from build123d import *

# Parameters (mm, degrees)
F0_W     = 50
F0_H     = 200
F1_DEPTH = 10
F2_R     = 3
F3_DEPTH = 25
F5_DEPTH = 25
F6_W     = 10
F6_H     = 10
F7_DEPTH = 10


with BuildPart() as f1:
    # F0 (on Front) → F1 (new body)
    with BuildSketch(Plane.XZ):
        Rectangle(F0_W, F0_H)
    extrude(amount=F1_DEPTH)

    # F2 (on face) → F3 (cut)
    with BuildSketch(Plane.XZ.offset(10)):
        with Locations((0, -25)):
            Circle(F2_R)
    extrude(amount=-F3_DEPTH, mode=Mode.SUBTRACT)

    # F4 (on face) → F5 (cut)
    with BuildSketch(Plane.XZ.offset(10)):
        with BuildLine():
            Line((10, 105), (-10, 105))
            Line((-10, 105), (-10, 75))
            ThreePointArc((-10, 75), (-8.5, 73.5), (-7, 75))
            Line((-7, 75), (7, 75))
            ThreePointArc((7, 75), (8.5, 73.5), (10, 75))
            Line((10, 75), (10, 105))
        make_face()
    extrude(amount=-F5_DEPTH, mode=Mode.SUBTRACT)

    # F6 (on face) → F7 (join)
    with BuildSketch(Plane.XZ.offset(10)):
        with Locations((-30, 65)):
            Rectangle(F6_W, F6_H)
        with Locations((30, 65)):
            Rectangle(F6_W, F6_H)
        with Locations((-30, -5)):
            Rectangle(F6_W, F6_H)
        with Locations((30, -5)):
            Rectangle(F6_W, F6_H)
    extrude(amount=-F7_DEPTH)


solid = f1.part
Source: CAD feature listing. Evaluate the final solid. Frame: model axes, mm. A direction names the side the tool comes from. Coordinates: 2 decimals unless noted, no trailing zeros. Loops run counter-clockwise (first coordinate to the right, second up) from the corner with the lowest first, then second, coordinate; pieces in that order, holes last. Notation, with made-up numbers: (5.25, 45.25) -> (16.25, 45.25) arc R22 cw to (16.25, 64.25) -> close; hole circle Ø7 at (85, 7.5). An arc over 180 degrees is marked (long way). Answer in a Markdown table with one row per item. Add a question column.
Q1. Ray query, line 1 along Z through (x, y) = (0, -7.25); line 2 along X through (y, z) = (-3.5, 82); line 3 along X through (y, z) = (-3, -48). Return the intervals inside material, ascending.
Q2. Section A-A on y = -1.5. Return the cut outline in (x, z).
Q3. Section B-B on x = 0. Return the cut outline in (y, z), and give its area (3 significant figures).
Q4. Contact query for flat-ended pins moving along their axis: pin 1 Ø3 at (x, y) = (-30.5, -5) entering from -Z; pin 2 Ø1 at (y, z) = (-2.5, 44.5) entering from +X; pin 3 Ø5 at (x, z) = (0, -25) entering from +Y; pin 4 Ø5 at (y, z) = (-3, 81.5) entering from -X. Output: stop coordinate, or through.
Q5. Reachability of faces 5 (the face through (25, -5, -56)), 6 (the face through (-30, -5, 70)), 7 (the face through (30, -5, 0)), 8 (the face through (0, -5, 75)) from +Z, -Z, +X, -X, +Y, -Y: full face, straight path, thin tool, end or side. Return the list, or none.
Q6. Section D-D on z = 5.5. Return the cut outline in (x, y), and give its area (3 significant figures).
Q7. Section C-C on z = -25. Return the cut outline in (x, y), and give its area (3 significant figures).
Q8. Pull-direction query (Z, two-part tool) for faces 1 (the face through (0, -5, -100)), 2 (the face through (-30, -5, 60)), 3 (the face through (17, -5, 100)), 4 (the face through (10, -5, 87)); classes: pulls with the +Z half, pulls with the -Z half, needs draft (parallel to the pull), parting line crosses it, or undercut.
Computed values:
| question | item | result |
|---|---|---|
| 1 | line 1 | z = -100 to -28, -22 to 75 |
| 1 | line 2 | x = -25 to -10, 10 to 25 |
| 1 | line 3 | x = -25 to 25 |
| 2 | outline | (-35, -10) -> (-25, -10) -> (-25, -100) -> (25, -100) -> (25, -10) -> (35, -10) -> (35, 0) -> (25, 0) -> (25, 60) -> (35, 60) -> (35, 70) -> (25, 70) -> (25, 100) -> (10, 100) -> (10, 75) arc R1.5 cw to (7, 75) -> (-7, 75) arc R1.5 cw to (-10, 75) -> (-10, 100) -> (-25, 100) -> (-25, 70) -> (-35, 70) -> (-35, 60) -> (-25, 60) -> (-25, 0) -> (-35, 0) -> close; hole circle Ø6 at (0, -25) |
| 3 | outline | (-10, -100) -> (0, -100) -> (0, -28) -> (-10, -28) -> close; (-10, -22) -> (0, -22) -> (0, 75) -> (-10, 75) -> close |
| 3 | area | 1,690 mm^2 |
| 4 | pin 1 | stops at z = -10 |
| 4 | pin 2 | stops at x = 25 |
| 4 | pin 3 | passes through |
| 4 | pin 4 | stops at x = -25 |
| 5 | face 5 | -Z, +X, +Y, -Y |
| 5 | face 6 | +Z, -X, +Y, -Y |
| 5 | face 7 | +X, +Y, -Y |
| 5 | face 8 | +Z, +Y, -Y |
| 6 | outline | (-25, -10) -> (25, -10) -> (25, 0) -> (-25, 0) -> close |
| 6 | area | 500 mm^2 |
| 7 | outline | (-25, -10) -> (-3, -10) -> (-3, 0) -> (-25, 0) -> close; (3, -10) -> (25, -10) -> (25, 0) -> (3, 0) -> close |
| 7 | area | 440 mm^2 |
| 8 | face 1 | pulls with the -Z half |
| 8 | face 2 | undercut |
| 8 | face 3 | pulls with the +Z half |
| 8 | face 4 | needs draft |
